Can you work these out from the model? Positions are in its coordinate system, mm. Coordinates: 2 decimals unless noted, no trailing zeros. Write each loop counter-clockwise with the first axis right and the second up, starting at its lowest first coordinate (ties: lowest second). Pieces come first, ordered by that corner, then holes. Notation, with made-up numbers: M 74,72 L 117,72 A19 cw 117,101 Z; hole C -19.75,81.25 d4. An arc over 180 degrees is marked long. Use one line per item in the form item = value. Start each with the question number.
```python
from build123d import *

# Parameters (mm, degrees)
F1_DEPTH = 50.8
F3_D     = 6.604


with BuildPart() as f1:
    # F0 (on Front) → F1 (new body)
    with BuildSketch(Plane.XZ):
        with BuildLine():
            ThreePointArc((-7.7199247783, -24.1984041089), (-14.9845572279, 20.5090966326), (25.4, 0))
            ThreePointArc((25.4, 0), (20.5090966326, -14.9845572279), (7.7199247783, -24.1984041089))
            Line((7.7199247783, -24.1984041089), (20.5547984321, -24.1984041089))
            ThreePointArc((20.5547984321, -24.1984041089), (28.8155977746, -13.3313099465), (31.75, 0))
            ThreePointArc((31.75, 0), (-13.3313099465, 28.8155977746), (-20.5547984321, -24.1984041089))
            Line((-20.5547984321, -24.1984041089), (-7.7199247783, -24.1984041089))
        make_face()
        with BuildLine():
            ThreePointArc((7.7199247783, -24.1984041089), (0, -25.4), (-7.7199247783, -24.1984041089))
            Line((-7.7199247783, -24.1984041089), (-20.5547984321, -24.1984041089))
            ThreePointArc((-20.5547984321, -24.1984041089), (0, -31.75), (20.5547984321, -24.1984041089))
            Line((20.5547984321, -24.1984041089), (7.7199247783, -24.1984041089))
        make_face()
        with BuildLine():
            ThreePointArc((20.5547984321, -24.1984041089), (0, -31.75), (-20.5547984321, -24.1984041089))
            Line((-20.5547984321, -24.1984041089), (-38.1, -24.1984041089))
            Line((-38.1, -24.1984041089), (-38.1, -39.3015958911))
            Line((-38.1, -39.3015958911), (38.1, -39.3015958911))
            Line((38.1, -39.3015958911), (38.1, -24.1984041089))
            Line((38.1, -24.1984041089), (20.5547984321, -24.1984041089))
        make_face()
    extrude(amount=F1_DEPTH)

    # F3 (through all)
    with Locations(Plane(origin=(0, 0, -39.3015958911), x_dir=(1, 0, 0), z_dir=(0, 0, -1))):
        with Locations((-25.4, 25.4), (25.4, 25.4)):
            Hole(F3_D / 2)


solid = f1.part
```
1) Suppose I cut it at A-A on x = 0. Please give me the cut outline in (y, z), and give its area (3 significant figures).
2) Suppose I cut it at B-B on y = -16.5. Please give me the cut outline in (x, z).
3) Please list where these lines run through material, in increasing order: line 1 (Z direction, x = 0, y = -37); line 2 (Z direction, x = 23, y = -46.5); line 3 (X direction, y = -25, z = -32).
4) Will these pins go through, and if not, where does the flat tip stop? pin 1 Ø12 at (x, z) = (-14.5, 1.5) entering from -Y; pin 2 Ø7.5 at (x, y) = (-25.4, -25.4) entering from +Z; pin 3 Ø19.5 at (x, y) = (32, -18) entering from +Z; pin 4 Ø10.5 at (x, y) = (25.4, -25.4) entering from +Z.
5) Suppose I cut it at D-D on x = -24. Please give me the cut outline in (y, z), and give its area (3 significant figures).
6) If we mould it in two halves opening along X, with no side actions, what happens to faces 1 (the face through (-24.97, -28.674, -31.644)), 2 (the face through (38.1, -25, -32)), 3 (the face through (-1, -25, -39.302))? For each: +X half, -X half, draft (parallel to the pull), parting line (faces both ways), or undercut.
7) Suppose I cut it at C-C on z = 3. Please give me the cut outline in (x, y).
Computed values:
q1.outline = M -50.8,-39.3 L 0,-39.3 L 0,-25.4 L -50.8,-25.4 Z; M -50.8,25.4 L 0,25.4 L 0,31.75 L -50.8,31.75 Z
q1.area = 1,030 mm²
q2.outline = M -38.1,-39.3 L 38.1,-39.3 L 38.1,-24.2 L 20.55,-24.2 A31.75 ccw long -20.55,-24.2 L -38.1,-24.2 Z; hole C 0,0 d50.8
q3.line_1 = -39.3 to -25.4, 25.4 to 31.75
q3.line_2 = -39.3 to -24.2, -21.89 to -10.78, 10.78 to 21.89
q3.line_3 = -38.1 to -28.68, -22.12 to 22.12, 28.68 to 38.1
q4.pin_1 = through
q4.pin_2 = 23.22
q4.pin_3 = 22.65
q4.pin_4 = 24.54
q5.outline = M -50.8,-39.3 L -28.39,-39.3 L -28.39,-24.2 L -50.8,-24.2 Z; M -50.8,-20.79 L -28.39,-20.79 L -28.39,-8.32 L -50.8,-8.32 Z; M -50.8,8.32 L -28.39,8.32 L -28.39,20.79 L -50.8,20.79 Z; M -22.41,-39.3 L 0,-39.3 L 0,-24.2 L -22.41,-24.2 Z; M -22.41,-20.79 L 0,-20.79 L 0,-8.32 L -22.41,-8.32 Z; M -22.41,8.32 L 0,8.32 L 0,20.79 L -22.41,20.79 Z
q5.area = 1,790 mm²
q6.face_1 = undercut
q6.face_2 = +X half
q6.face_3 = draft
q7.outline = M -31.61,-50.8 L -25.22,-50.8 L -25.22,-28.7 A3.3 cw long -25.22,-22.1 L -25.22,0 L -31.61,0 Z; M 25.22,-50.8 L 31.61,-50.8 L 31.61,0 L 25.22,0 L 25.22,-22.1 A3.3 cw long 25.22,-28.7 Z
